from build123d import *

# Parameters (mm, degrees)
BASE_FLANGE1_DEPTH = 211
SKETCH2_R          = 8
EXTRUDE2_DEPTH     = 214.604031327
SKETCH3_R          = 1.75
EXTRUDE3_DEPTH     = 0.5
SKETCH4_R          = 1.75
EXTRUDE4_DEPTH     = 0.5


# Sheet-metal steps are written as plain solids
with BuildPart() as part:
    # Sketch1 → Base-Flange1 (new, symmetric)
    with BuildSketch(Plane.XY):
        with BuildLine():
            Line((4.055025352, 3.715746142), (0.430067214, 0.394083995))
            ThreePointArc((0.430067214, 0.394083995), (-0.03966104, 0.101988196), (-0.583318098, 0))
            Line((-0.583318098, 0), (-31, 0))
            ThreePointArc((-31, 0), (-32.5, -1.5), (-31, -3))
            Line((-31, -3), (-26, -3))
            Line((-26, -3), (-26, -3.5))
            Line((-26, -3.5), (-31, -3.5))
            ThreePointArc((-31, -3.5), (-33, -1.5), (-31, 0.5))
            Line((-31, 0.5), (-0.583318098, 0.5))
            ThreePointArc((-0.583318098, 0.5), (-0.220880059, 0.567992131), (0.09227211, 0.762722663))
            Line((0.09227211, 0.762722663), (3.717230249, 4.08438481))
            Line((3.717230249, 4.08438481), (4.055025352, 3.715746142))
        make_face()
    extrude(amount=BASE_FLANGE1_DEPTH, both=True)

    # Sketch2 → Extrude2 (cut, through all)
    with BuildSketch(Plane(origin=(0, 0, 0), x_dir=(1, 0, 0), z_dir=(0, 1, 0))):
        with Locations(Location((-14.883318098, 201, 0), (0, 0, 180))):
            Circle(SKETCH2_R)
        with Locations(Location((-14.883318098, -201, 0), (0, 0, 90))):
            Circle(SKETCH2_R)
    extrude(amount=EXTRUDE2_DEPTH, mode=Mode.SUBTRACT)

    # Sketch3 → Extrude3 (cut)
    with BuildSketch(Plane(origin=(0, 0.5, 0), x_dir=(1, 0, 0), z_dir=(0, 1, 0))):
        with Locations(Location((-14.883318098, 0, 0), (0, 0, 180))):
            Circle(SKETCH3_R)
    extrude(amount=-EXTRUDE3_DEPTH, mode=Mode.SUBTRACT)

    # Sketch4 → Extrude4 (cut)
    with BuildSketch(Plane(origin=(0, 0.5, 0), x_dir=(1, 0, 0), z_dir=(0, 1, 0))):
        with Locations(Location((-14.883318098, 184, 0), (0, 0, 180))):
            Circle(SKETCH4_R)
        with Locations((-14.883318098, -184)):
            Circle(SKETCH4_R)
    extrude(amount=-EXTRUDE4_DEPTH, mode=Mode.SUBTRACT)


solid = part.part
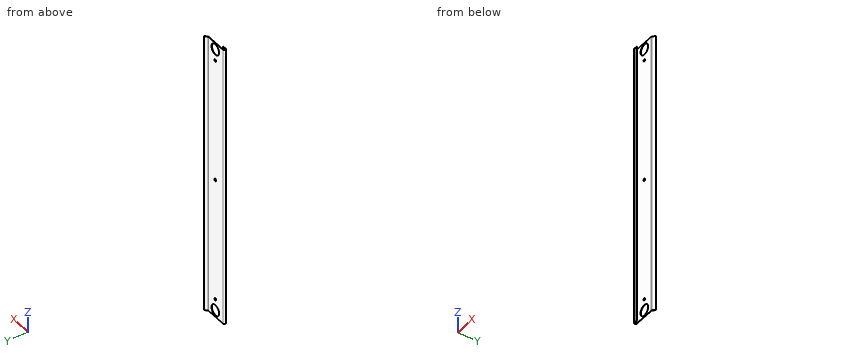
Build history of the part. All positions in model axes, mm. Coordinates: 2 decimals unless noted, no trailing zeros. Order: outer loops, then holes, each group sorted by start corner. A loop starts at its lowest first (then second) coordinate and runs counter-clockwise, first axis right, second up. Notation, with made-up numbers: (11.5, -37) - (55.5, -37) arc R32 cw to (55.5, -5) - close; hole circle Ø7 at (82.25, -5). An arc over 180 degrees is marked (long way). Write item = value, one per line. Start each with the question number.
1) Flat gauge pins, fed straight in: pin 1 Ø4 at (x, z) = (-28, 26.5) entering from +Y; pin 2 Ø0.6 at (y, z) = (-3.5, -105) entering from +X. Where does each tip first touch, or does it go through?
2) Saw through at C-C on y = -1.5. Write the cut outline in (x, z).
3) Saw through at B-B on z = 73.5. Write the cut outline in (x, y), then the cut area to 3 significant figures.
4) Saw through at A-A on z = 201. Write the cut outline in (x, y).
5) Wall check: line 1 along Y through (x, z) = (-6, 180); line 2 along X through (y, z) = (0.75, -34); line 3 along X through (y, z) = (0.25, -201). Give the ranges that are in metal, low to high. Write a range as from..to.
From the geometry:
q1.pin_1 = 0.5
q1.pin_2 = -26
q2.outline = (-33, -211) - (-32.5, -211) - (-32.5, 211) - (-33, 211) - close
q3.outline = (-31, -3.5) - (-26, -3.5) - (-26, -3) - (-31, -3) arc R1.5 cw to (-31, 0) - (-0.58, 0) arc R1.5 ccw to (0.43, 0.39) - (4.06, 3.72) - (3.72, 4.08) - (0.09, 0.76) arc R1 cw to (-0.58, 0.5) - (-31, 0.5) arc R2 ccw to start
q3.area = 23.4 mm^2
q4.outline = (-31, -3.5) - (-26, -3.5) - (-26, -3) - (-31, -3) arc R1.5 cw to (-31, 0) - (-22.88, 0) - (-22.88, 0.5) - (-31, 0.5) arc R2 ccw to start; (-6.88, 0) - (-0.58, 0) arc R1.5 ccw to (0.43, 0.39) - (4.06, 3.72) - (3.72, 4.08) - (0.09, 0.76) arc R1 cw to (-0.58, 0.5) - (-6.88, 0.5) - close
q5.line_1 = 0..0.5
q5.line_2 = 0.08..0.82
q5.line_3 = -31.97..-22.88, -6.88..0.25
